The listing builds one solid part. Answer for the finished solid, in the listing's coordinates (mm). Coordinates: 2 decimals unless noted, no trailing zeros. Write each loop counter-clockwise with the first axis right and the second up, starting at its lowest first coordinate (ties: lowest second). Pieces come first, ordered by that corner, then holes.
from build123d import *

# Parameters (mm, degrees)
SKETCH1_W      = 26
SKETCH1_H      = 12
EXTRUDE1_DEPTH = 1.5
SKETCH2_R      = 1.63
EXTRUDE2_DEPTH = 2.5


with BuildPart() as part:
    # Sketch1 → Extrude1 (new body)
    with BuildSketch(Plane.XY):
        with Locations((-13, 6)):
            Rectangle(SKETCH1_W, SKETCH1_H)
    extrude(amount=-EXTRUDE1_DEPTH)

    # Sketch2 → Extrude2 (cut, through all)
    with BuildSketch(Plane.XY):
        with Locations((-12.9924, 2.5)):
            Circle(SKETCH2_R)
        with Locations((-2.9848, 2.5)):
            Circle(SKETCH2_R)
        with Locations(Location((-2.9848, 9.5, 0), (0, 0, 180))):  # turned: the seam where the file's is
            Circle(SKETCH2_R)
        with Locations(Location((-12.9924, 9.5, 0), (0, 0, 180))):  # turned: the seam where the file's is
            Circle(SKETCH2_R)
        with Locations((-23, 2.5)):
            Circle(SKETCH2_R)
        with Locations(Location((-23, 9.5, 0), (0, 0, 180))):  # turned: the seam where the file's is
            Circle(SKETCH2_R)
    extrude(amount=-EXTRUDE2_DEPTH, mode=Mode.SUBTRACT)


solid = part.part
Q1. Determine the mould class of faces 1 (the face through (-13, 12, -1)), 2 (the face through (0, 6, -1)), 3 (the face through (-2.773, 7.884, -0.74)) for opening direction Y: released by +Y, released by -Y, zero draft, split by the parting line, or undercut.
Answers below:
face 1: released by +Y
face 2: zero draft
face 3: undercut
Q2. The part is cut by section D-D, the plane y = 1.5. Write down the section's boundary in (x, z).
Answers below:
outline: (-26, -1.5) - (-24.29, -1.5) - (-24.29, 0) - (-26, 0) - close; (-21.71, -1.5) - (-14.28, -1.5) - (-14.28, 0) - (-21.71, 0) - close; (-11.71, -1.5) - (-4.27, -1.5) - (-4.27, 0) - (-11.71, 0) - close; (-1.7, -1.5) - (0, -1.5) - (0, 0) - (-1.7, 0) - close
Q3. Find the intervals of material crossed by probe 1 along X at (y, z) = (9.5, -0.9); probe 2 along Y at (x, z) = (-23, -1.15); probe 3 along X at (y, z) = (8.75, -0.85), in increasing order.
Answers below:
probe 1: x = -26 to -24.63, -21.37 to -14.62, -11.36 to -4.61, -1.35 to 0
probe 2: y = 0 to 0.87, 4.13 to 7.87, 11.13 to 12
probe 3: x = -26 to -24.45, -21.55 to -14.44, -11.55 to -4.43, -1.54 to 0
Q4. The part is cut by section A-A, the plane x = -23. Write down the section's boundary in (y, z), then the cut area to 3 significant figures.
Answers below:
outline: (0, -1.5) - (0.87, -1.5) - (0.87, 0) - (0, 0) - close; (4.13, -1.5) - (7.87, -1.5) - (7.87, 0) - (4.13, 0) - close; (11.13, -1.5) - (12, -1.5) - (12, 0) - (11.13, 0) - close
area: 8.22 mm2
Q5. The part is cut by section B-B, the plane z = -0.7. Write down the section's boundary in (x, y), then the cut area to 3 significant figures.
Answers below:
outline: (-26, 0) - (0, 0) - (0, 12) - (-26, 12) - close; hole circle Ø3.26 at (-23, 2.5); hole circle Ø3.26 at (-23, 9.5); hole circle Ø3.26 at (-12.99, 2.5); hole circle Ø3.26 at (-12.99, 9.5); hole circle Ø3.26 at (-2.98, 2.5); hole circle Ø3.26 at (-2.98, 9.5)
area: 262 mm2
Q6. The part is cut by section C-C, the plane y = 9.5. Write down the section's boundary in (x, z), then the cut area to 3 significant figures.
Answers below:
outline: (-26, -1.5) - (-24.63, -1.5) - (-24.63, 0) - (-26, 0) - close; (-21.37, -1.5) - (-14.62, -1.5) - (-14.62, 0) - (-21.37, 0) - close; (-11.36, -1.5) - (-4.61, -1.5) - (-4.61, 0) - (-11.36, 0) - close; (-1.35, -1.5) - (0, -1.5) - (0, 0) - (-1.35, 0) - close
area: 24.3 mm2
